```python
from build123d import *

# Parameters (mm, degrees)
F0_R     = 5.3
F0_R_2   = 3.85
F1_DEPTH = 2
F2_DEPTH = 6.5
F3_DEPTH = 4
F4_R     = 0.95
F5_DEPTH = 25.4
F6_R     = 1


with BuildPart() as f1:
    # F0 (on Front) → F1 (new body)
    with BuildSketch(Plane.XZ):
        Circle(F0_R)
        Circle(F0_R_2, mode=Mode.SUBTRACT)
    extrude(amount=F1_DEPTH)

    # F0 (on Front) → F2 (join)
    with BuildSketch(Plane.XZ):
        with BuildLine():
            ThreePointArc((1.6268819186, -6.6025188545), (5.352709387, -4.1938648308), (6.8, 3.00667e-05))
            ThreePointArc((6.8, 3.00667e-05), (-3.00667e-05, 6.8), (-6.8, -3.00667e-05))
            ThreePointArc((-6.8, -3.00667e-05), (-5.4303317767, -4.0928592445), (-1.8731180814, -6.5369280747))
            ThreePointArc((-1.8731180814, -6.5369280747), (-0.1274111438, -6.7988062483), (1.6268819186, -6.6025188545))
        make_face()
        Circle(F0_R, mode=Mode.SUBTRACT)
    extrude(amount=F2_DEPTH)

    # F0 (on Front) → F3 (join)
    with BuildSketch(Plane.XZ):
        with BuildLine():
            Line((1.6268819186, -10.0241614027), (1.6268819186, -6.6025188544))
            ThreePointArc((1.6268819186, -6.6025188545), (-0.1274111438, -6.7988062483), (-1.8731180814, -6.5369280747))
            Line((-1.8731180814, -6.5369280746), (-1.8731180814, -10.0241614027))
            Line((-1.8731180814, -10.0241614027), (1.6268819186, -10.0241614027))
        make_face()
    extrude(amount=F3_DEPTH)

    # F4 (on face) → F5 (cut)
    with BuildSketch(Plane.YZ.offset(1.6268819186)):
        with Locations((-2.055265424, -8.0741614027)):
            Circle(F4_R)
    extrude(amount=-F5_DEPTH, mode=Mode.SUBTRACT)

    # F6
    f6_edges = [f1.edges().sort_by_distance(p)[0] for p in [
        (1.626882, -2, -10.024161),
        (-1.873118, -2, -10.024161),
        (-0.123118, -4, -10.024161),
    ]]
    fillet(f6_edges, radius=F6_R)


solid = f1.part
```
Source: CAD feature listing. Evaluate the final solid. Frame: model axes, mm. A direction names the side the tool comes from. Give positions to 0.01 mm unless a question says otherwise; leave off trailing zeros. Order: outer loops, then holes, each group sorted by start corner. A loop starts at its lowest first (then second) coordinate and runs counter-clockwise, first axis right, second up.
(1) Section query C-C (y = -5.75). Return the cut outline in (x, z).
(2) Contact query for flat-ended pins moving along their axis: P1, Ø2, axis at x = -0.5, z = -7.5, coming from the -Y side; P2, Ø1.2, axis at y = -2, z = -7.5, coming from the +X side; P3, Ø3, axis at y = -2, z = -6, coming from the -X side; P4, Ø1.5, axis at y = -3, z = -1, coming from the +X side. Output: stop coordinate, or through.
(3) Section query B-B (z = 1). Return the cut outline in (x, y), plus the area to 3 significant figures.
(4) Pull-direction query (X, two-part tool) for faces 1 (the face through (4, -2, 2)), 2 (the face through (-1.873, -2, -6.9)), 3 (the face through (-4, -6.5, -4)); classes: +X half, -X half, draft (parallel to the pull), parting line (faces both ways), or undercut.
(5) Section query D-D (x = 3.5). Return the cut outline in (y, z), plus the area to 3 significant figures.
(6) Section query A-A (x = 0). Return the cut outline in (y, z).
(7) Access query for faces 4 (the face through (1.627, -1.5, -7)), 5 (the face through (-0.1, -3.81, -9.61)), 6 (the face through (4.896, -4.219, -2.03)). Directions: +Z, -Z, +X, -X, +Y, -Y. A direction counts if a zero-diameter tool reaches every point of the face in a straight line with its end or side. Return the directions, or none.
(8) Material intervals for line 1 along Z through (x, y) = (0, -3.1); line 2 along Y through (x, z) = (-1, 4.75); line 3 along X through (y, z) = (-0.25, 1), sorted ascending.
Outcome:
1. outline: circle Ø13.6 at (0, 0); hole circle Ø10.6 at (0, 0)
2. P1: stops at y = -6.5
2. P2: stops at x = 1.63
2. P3: stops at x = -5.1
2. P4: stops at x = 6.8
3. outline: (-6.73, -6.5) - (-5.2, -6.5) - (-5.2, -2) - (-3.72, -2) - (-3.72, 0) - (-6.73, 0) - close; (3.72, -2) - (5.2, -2) - (5.2, -6.5) - (6.73, -6.5) - (6.73, 0) - (3.72, 0) - close
3. area: 25.7 mm2
4. face 1: undercut
4. face 2: -X half
4. face 3: draft
5. outline: (-6.5, -5.83) - (0, -5.83) - (0, -1.6) - (-2, -1.6) - (-2, -3.98) - (-6.5, -3.98) - close; (-6.5, 3.98) - (-2, 3.98) - (-2, 1.6) - (0, 1.6) - (0, 5.83) - (-6.5, 5.83) - close
5. area: 33.6 mm2
6. outline: (-6.5, -6.8) - (-4, -6.8) - (-4, -9.02) arc R1 ccw to (-3, -10.02) - (0, -10.02) - (0, -3.85) - (-2, -3.85) - (-2, -5.3) - (-6.5, -5.3) - close; (-6.5, 5.3) - (-2, 5.3) - (-2, 3.85) - (0, 3.85) - (0, 6.8) - (-6.5, 6.8) - close; hole circle Ø1.9 at (-2.06, -8.07)
7. face 4: -Z, +X, +Y, -Y
7. face 5: -Z, +X, -X, -Y
7. face 6: -Y
8. line 1: z = -10.02 to -5.3, 5.3 to 6.8
8. line 2: y = -2 to 0
8. line 3: x = -6.73 to -3.72, 3.72 to 6.73
